from build123d import *

# Parameters (mm, degrees)
SKETCH1_R           = 1.5
BOSS_EXTRUDE1_DEPTH = 5
SKETCH2_R           = 15
BOSS_EXTRUDE2_DEPTH = 15
SKETCH3_R           = 30
BOSS_EXTRUDE3_DEPTH = 35
SKETCH6_R           = 7.5
BOSS_EXTRUDE5_DEPTH = 60
CHAMFER2_SIZE       = 2


with BuildPart() as part:
    # Sketch1 → Boss-Extrude1 (new body)
    with BuildSketch(Plane.XY):
        with BuildLine():
            Line((-3, 38), (-3, 34.871191548))
            ThreePointArc((-3, 34.871191548), (-35, 0), (-3, -34.871191548))
            Line((-3, -34.871191548), (-3, -38))
            ThreePointArc((-3, -38), (0, -41), (3, -38))
            Line((3, -38), (3, -34.871191548))
            ThreePointArc((3, -34.871191548), (35, 0), (3, 34.871191548))
            Line((3, 34.871191548), (3, 38))
            ThreePointArc((3, 38), (0, 41), (-3, 38))
        make_face()
        with Locations((0, 38)):
            Circle(SKETCH1_R, mode=Mode.SUBTRACT)
        with Locations(Location((0, -38, 0), (0, 0, 180))):
            Circle(SKETCH1_R, mode=Mode.SUBTRACT)
    extrude(amount=-BOSS_EXTRUDE1_DEPTH)

    # Sketch2 → Boss-Extrude2 (add)
    with BuildSketch(Plane.XY):
        with Locations(Location((0, 0, 0), (0, 0, 180))):
            Circle(SKETCH2_R)
    extrude(amount=BOSS_EXTRUDE2_DEPTH)

    # Sketch3 → Boss-Extrude3 (add)
    with BuildSketch(Plane(origin=(0, 0, -5), x_dir=(-1, 0, 0), z_dir=(0, 0, -1))):
        Circle(SKETCH3_R)
    extrude(amount=BOSS_EXTRUDE3_DEPTH)

    # Loft1: read off the stored shape, not the designer's step
    # Loft1: loft between two sections, ruled curve by curve
    loft1_from = [
        Edge.make_bspline([(4.132315812, 9.106259717, -40), (22.344835246, 0.841628092, -40), (14.080203621, -17.370891341, -40), (-4.132315812, -9.106259717, -40), (-22.344835246, -0.841628092, -40), (-14.080203621, 17.370891341, -40), (4.132315812, 9.106259717, -40)], [0, 0, 0, 0, 0.5, 0.5, 0.5, 1, 1, 1, 1], 3, [1, 0.333333333, 0.333333333, 1, 0.333333333, 0.333333333, 1]),
    ]
    loft1_to = [
        Edge.make_bspline([(5.329891047, 5.276576677, -47), (15.8830444, -5.383205418, -47), (5.223262306, -15.936358771, -47), (-5.329891047, -5.276576677, -47), (-15.8830444, 5.383205418, -47), (-5.223262306, 15.936358771, -47), (5.329891047, 5.276576677, -47)], [0, 0, 0, 0, 0.5, 0.5, 0.5, 1, 1, 1, 1], 3, [1, 0.333333333, 0.333333333, 1, 0.333333333, 0.333333333, 1]),
    ]
    loft1 = Solid(Shell([*[Face.make_surface_from_curves(loft1_from[k], loft1_to[k]) for k in range(1)], Face(Wire(loft1_from)), Face(Wire(loft1_to))]))
    add(loft1)

    # Sketch6 → Boss-Extrude5 (add)
    with BuildSketch(Plane(origin=(0, 0, -47), x_dir=(-1, 0, 0), z_dir=(0, 0, -1))):
        with Locations(Location((0, 0, 0), (0, 0, 135.288))):
            Circle(SKETCH6_R)
    extrude(amount=BOSS_EXTRUDE5_DEPTH)

    # Chamfer2
    chamfer2_edges = [part.edges().sort_by_distance(p)[0] for p in [
        (-5.329891047, -5.276576677, -107),
    ]]
    chamfer(chamfer2_edges, length=CHAMFER2_SIZE)


solid = part.part
The listing builds one solid part. Answer for the finished solid, in the listing's coordinates (mm). A direction names the side the tool comes from. Give positions to 0.01 mm unless a question says otherwise; leave off trailing zeros. Write each loop counter-clockwise with the first axis right and the second up, starting at its lowest first coordinate (ties: lowest second). Pieces come first, ordered by that corner, then holes.
Item 1: Section A-A, the plane x = 0 is taken. Count the separate pieces of the cut face and the enclosed holes in it, plus the area to 3 significant figures.
Item 2: Determine the mould class of faces 4 (the cylindrical face through (-0.325, 36.536, -2.465)), 5 (the flat face through (3, -36, -2)), 6 (the cylindrical face through (-34.992, 0.728, -2.465)) for opening direction Y: released by +Y, released by -Y, zero draft, split by the parting line, or undercut.
Item 3: Which of the six approach directions +Z, -Z, +X, -X, +Y, -Y give full straight-line access (tool end or side, diameter ignored) to faces 1 (the cylindrical face through (-8.06, -12.65, 7.4)), 2 (the cylindrical face through (29.97, 1.32, -22.26)), 3 (the flat face through (-3, 36, -2))?
Item 4: Find the intervals of material crossed by line 1 along Y through (x, z) = (0, -3.3); line 2 along X through (y, z) = (-38, -1.45); line 3 along Z through (x, y) = (17.5, -25), in increasing order.
Item 5: Flat-ended cylindrical pins translate along their axes: P1, Ø12, axis at x = -2, y = -28, coming from the +Z side; P2, Ø4, axis at y = 20, z = -4, coming from the +X side; P3, Ø1.6, axis at y = -37, z = -1.5, coming from the -X side. Find the tip coordinate at first contact, or state that the pin passes through.
Item 6: Section D-D, the plane x = -26 is taken. Write down the section's boundary in (y, z), plus the area to 3 significant figures.
Item 7: Section C-C, the plane z = -18 is taken. Write down the section's boundary in (x, y).
Item 8: Section B-B, the plane y = 27.5 is taken. Write down the section's boundary in (x, z).
Completed:
1. separate pieces: 3
1. enclosed holes: 0
1. area: 3,950 mm2
2. face 4: undercut
2. face 5: zero draft
2. face 6: split by the parting line
3. face 1: +Z
3. face 2: -Z
3. face 3: +Z, -Z, -X, +Y
4. line 1: y = -41 to -39.5, -36.5 to 36.5, 39.5 to 41
4. line 2: x = -3 to -1.5, 1.5 to 3
4. line 3: z = -5 to 0
5. P1: stops at z = 0
5. P2: stops at x = 30.02
5. P3: stops at x = -3
6. outline: (-23.43, -5) - (-14.97, -5) - (-14.97, -40) - (14.97, -40) - (14.97, -5) - (23.43, -5) - (23.43, 0) - (-23.43, 0) - close
6. area: 1,280 mm2
7. outline: circle Ø60 at (0, 0)
8. outline: (-21.65, -5) - (-11.99, -5) - (-11.99, -40) - (11.99, -40) - (11.99, -5) - (21.65, -5) - (21.65, 0) - (-21.65, 0) - close
